from build123d import *

# Parameters (mm, degrees)
F0_W          = 500
F0_H          = 120
F0_R          = 30
F1_DEPTH      = 25
F2_R          = 45
F3_DEPTH      = 40
F3_DEPTH_BACK = 90
F4_SIZE       = 90
F5_R          = 250


with BuildPart() as f1:
    # F0 (on Top) → F1 (new body, symmetric)
    with BuildSketch(Plane.XY):
        Rectangle(F0_W, F0_H)
        with Locations((-150, 0)):
            Circle(F0_R, mode=Mode.SUBTRACT)
        with Locations((150, 0)):
            Circle(F0_R, mode=Mode.SUBTRACT)
    extrude(amount=F1_DEPTH, both=True)

    # F2 (on face) → F3 (join, two sides)
    with BuildSketch(Plane.XY.offset(25)) as f3_sk:
        Circle(F2_R)
    extrude(amount=F3_DEPTH)
    extrude(f3_sk.sketch, amount=-F3_DEPTH_BACK)

    # F4
    f4_edges = [f1.edges().sort_by_distance(p)[0] for p in [
        (-250, -60, 0),
        (250, 60, 0),
    ]]
    chamfer(f4_edges, length=F4_SIZE)

    # F5
    f5_edges = [f1.edges().sort_by_distance(p)[0] for p in [
        (-160, -60, 0),
        (160, 60, 0),
    ]]
    fillet(f5_edges, radius=F5_R)


solid = f1.part
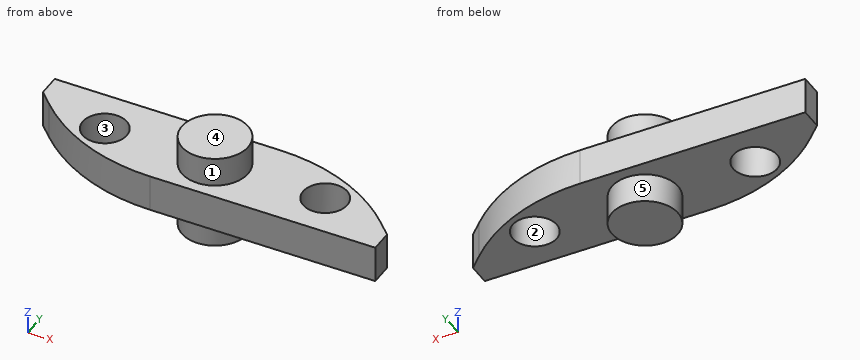
Can you work these out from the model? Positions are in its coordinate system, mm. Face numbers are marked on the shaded views. A direction names the side the tool comes from. Coordinates: 2 decimals unless noted, no trailing zeros. Write each loop counter-clockwise with the first axis right and the second up, starting at its lowest first coordinate (ties: lowest second). Pieces come first, ordered by that corner, then holes.
Q1. If we mould it in two halves opening along X, with no side actions, what happens to the marked faces 3, 4 and 5? For each: +X half, -X half, draft (parallel to the pull), parting line (faces both ways), or undercut.
Results found:
face 3: undercut
face 4: draft
face 5: parting line
Q2. Imagine slicing it at D-D, the plane x = 150. List the corners of the cut face in (y, z) for me.
Results found:
outline: (-60, -25) - (-30, -25) - (-30, 25) - (-60, 25) - close; (30, -25) - (41.84, -25) - (41.84, 25) - (30, 25) - close
Q3. Imagine slicing it at C-C, the plane x = 0. List the corners of the cut face in (y, z) for me.
Results found:
outline: (-60, -25) - (-45, -25) - (-45, -65) - (45, -65) - (45, -25) - (60, -25) - (60, 25) - (45, 25) - (45, 65) - (-45, 65) - (-45, 25) - (-60, 25) - close
Q4. Imagine slicing it at B-B, the plane y = 0. List the corners of the cut face in (x, z) for me, plus the area to 3 significant figures.
Results found:
outline: (-218.93, -25) - (-180, -25) - (-180, 25) - (-218.93, 25) - close; (-120, -25) - (-45, -25) - (-45, -65) - (45, -65) - (45, -25) - (120, -25) - (120, 25) - (45, 25) - (45, 65) - (-45, 65) - (-45, 25) - (-120, 25) - close; (180, -25) - (218.93, -25) - (218.93, 25) - (180, 25) - close
area: 23,100 mm2
Q5. Which directions (+Z, -Z, +X, -X, +Y, -Y) give clear straight access to the entire face, cutting with the end or side of a thin tool? Please do the marked faces 1 and 2.
Results found:
face 1: +Z
face 2: +Z, -Z
Q6. For P1, Ø1.5, axis at y = -22, z = 42.5, coming from the +X side; P2, Ø1, axis at x = -147.5, z = 24, coming from the -Y side; P3, Ø1.5, axis at x = -30.5, z = 33, coming from the +Y side, each with a flat end and sliding along its axis, tell me the tip position at first contact or that it passes through.
Results found:
P1: stops at x = 39.67
P2: stops at y = -43.02
P3: stops at y = 33.76
Q7. Imagine slicing it at A-A, the plane z = 2.5. List the corners of the cut face in (x, y) for me.
Results found:
outline: (-250, 30) - (-233.22, 13.22) arc R250 ccw to (-56.45, -60) - (250, -60) - (250, -30) - (233.22, -13.22) arc R250 ccw to (56.45, 60) - (-250, 60) - close; hole circle Ø60 at (-150, 0); hole circle Ø60 at (150, 0)
Q8. Please list where these lines run through material, in increasing order: L1, parallel to X at y = -2.5, z = -6; L2, parallel to X at y = -18, z = 24; L3, parallel to Z at x = -154, y = 33.5.
Results found:
L1: x = -215.96 to -179.9, -120.1 to 120.1, 179.9 to 221.81
L2: x = -195.14 to -174, -126 to 126, 174 to 238
L3: z = -25 to 25
